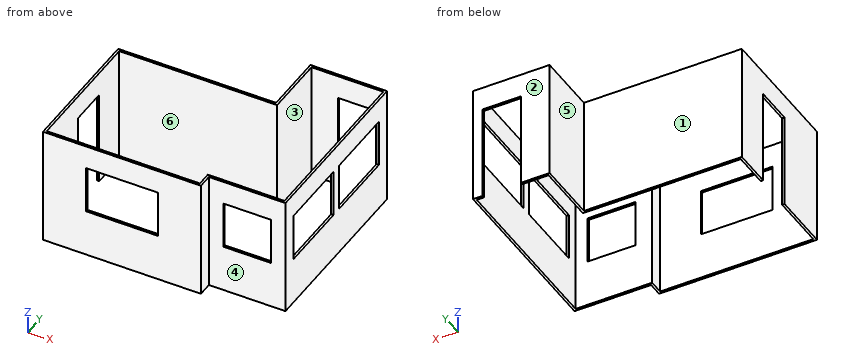
from build123d import *

# Parameters (mm, degrees)
F1_DEPTH  = 63.5
F2_W      = 38.1
F2_H      = 25.4
F3_DEPTH  = 1.27
F4_W      = 25.4
F4_H      = 25.4
F5_DEPTH  = 1.27
F6_W      = 38.1
F6_H      = 25.4
F7_DEPTH  = 1.27
F8_W      = 20.32
F8_H      = 50.8
F9_DEPTH  = 1.27
F10_W     = 20.32
F10_H     = 50.8
F11_DEPTH = 1.27


with BuildPart() as f1:
    # F0 (on Top) → F1 (new body)
    with BuildSketch(Plane.XY):
        Polygon((0, 32.766), (0, 0), (-83.82, 0), (-83.82, -71.628), (0, -71.628), (0, -64.008), (40.64, -64.008), (40.64, 32.766), align=None)
        Polygon((1.27, -1.27), (1.27, 31.496), (39.37, 31.496), (39.37, -62.738), (-1.27, -62.738), (-1.27, -70.358), (-82.55, -70.358), (-82.55, -1.27), align=None, mode=Mode.SUBTRACT)
    extrude(amount=F1_DEPTH)

    # F2 (on face) → F3 (cut)
    with BuildSketch(Plane.XZ.offset(71.628)):
        with Locations((-41.91, 38.1)):
            Rectangle(F2_W, F2_H)
    extrude(amount=-F3_DEPTH, mode=Mode.SUBTRACT)

    # F4 (on face) → F5 (cut)
    with BuildSketch(Plane.XZ.offset(64.008)):
        with Locations((20.32, 38.1)):
            Rectangle(F4_W, F4_H)
    extrude(amount=-F5_DEPTH, mode=Mode.SUBTRACT)

    # F6 (on face) → F7 (cut)
    with BuildSketch(Plane.YZ.offset(40.64)):
        with Locations((-37.338, 38.1)):
            Rectangle(F6_W, F6_H)
        with Locations((6.096, 38.1)):
            Rectangle(F6_W, F6_H)
    extrude(amount=-F7_DEPTH, mode=Mode.SUBTRACT)

    # F8 (on face) → F9 (cut)
    with BuildSketch(Plane(origin=(0, 32.766, 0), x_dir=(-1, 0, 0), z_dir=(0, 1, 0))):
        with Locations((-25.4, 25.4)):
            Rectangle(F8_W, F8_H)
    extrude(amount=-F9_DEPTH, mode=Mode.SUBTRACT)

    # F10 (on face) → F11 (cut)
    with BuildSketch(Plane(origin=(-83.82, 0, 0), x_dir=(0, -1, 0), z_dir=(-1, 0, 0))):
        with Locations((30.48, 25.4)):
            Rectangle(F10_W, F10_H)
    extrude(amount=-F11_DEPTH, mode=Mode.SUBTRACT)


solid = f1.part
Check sheet for the modelled part. Datum: model origin and axes. Units: mm. Face numbers are marked on the shaded views. A direction names the side the tool comes from. Give positions to 0.01 mm unless a question says otherwise; leave off trailing zeros. Write each loop counter-clockwise with the first axis right and the second up, starting at its lowest first coordinate (ties: lowest second). Pieces come first, ordered by that corner, then holes. Notation, with made-up numbers: (17.25, -32) -> (43.25, -32) arc R7 ccw to (43.25, -21) -> close; hole circle Ø1 at (84, 31). An arc over 180 degrees is marked (long way). Use one line per item in the form item = value. Start each with the question number.
1. Go/stop test with flat-tipped pins: P1, Ø16.5, axis at y = 9.5, z = 36.5, coming from the -X side; P2, Ø8, axis at y = -24.5, z = 31.5, coming from the +X side; P3, Ø19, axis at x = -45.5, z = 28.5, coming from the -Y side; P4, Ø11.5, axis at x = 20, z = 16, coming from the -Y side. Record where each tip stops, or that it passes through.
2. Section check D-D (x = -15.5). Record the cut outline in (y, z).
3. Access from +Z, -Z, +X, -X, +Y, -Y to the whole of each face (thin tool, end or side, straight path). Record for the marked faces 1, 2 and 3.
4. Mould release check, pull along X, two halves, no side actions. Record for the marked faces 4, 5 and 6: pulls with the +X half, pulls with the -X half, needs draft (parallel to the pull), parting line crosses it, or undercut.
5. Section check C-C (z = 22.5). Record the cut outline in (x, y).
6. Thickness scan on line 1 along Y through (x, z) = (-63.5, 29.5); line 2 along X through (y, z) = (20.5, 61.5); line 3 along Y through (x, z) = (4, 4.5). Record the ranges inside material, lowest first. Write a range as from..to.
7. Section check B-B (x = -56). Record the cut outline in (y, z), and give its area (3 significant figures).
8. Section check A-A (y = -26.5). Record the cut outline in (x, z), and give its area (3 significant figures).
Conclusion:
q1.P1 = 0
q1.P2 = through
q1.P3 = -71.63
q1.P4 = -64.01
q2.outline = (-71.63, 0) -> (-70.36, 0) -> (-70.36, 63.5) -> (-71.63, 63.5) -> close; (-1.27, 0) -> (0, 0) -> (0, 63.5) -> (-1.27, 63.5) -> close
q3.face_1 = +Z, -Z, -X, +Y
q3.face_2 = +Z, -Z, +X, -X, +Y
q3.face_3 = +Z, -Z
q4.face_4 = needs draft
q4.face_5 = pulls with the -X half
q4.face_6 = undercut
q5.outline = (-83.82, -71.63) -> (0, -71.63) -> (0, -64.01) -> (40.64, -64.01) -> (40.64, 32.77) -> (35.56, 32.77) -> (35.56, 31.5) -> (39.37, 31.5) -> (39.37, -62.74) -> (-1.27, -62.74) -> (-1.27, -70.36) -> (-82.55, -70.36) -> (-82.55, -40.64) -> (-83.82, -40.64) -> close; (-83.82, -20.32) -> (-82.55, -20.32) -> (-82.55, -1.27) -> (1.27, -1.27) -> (1.27, 31.5) -> (15.24, 31.5) -> (15.24, 32.77) -> (0, 32.77) -> (0, 0) -> (-83.82, 0) -> close
q6.line_1 = -71.63..-70.36, -1.27..0
q6.line_2 = 0..1.27, 39.37..40.64
q6.line_3 = -64.01..-62.74, 31.5..32.77
q7.outline = (-71.63, 0) -> (-70.36, 0) -> (-70.36, 25.4) -> (-71.63, 25.4) -> close; (-71.63, 50.8) -> (-70.36, 50.8) -> (-70.36, 63.5) -> (-71.63, 63.5) -> close; (-1.27, 0) -> (0, 0) -> (0, 63.5) -> (-1.27, 63.5) -> close
q7.area = 129 mm²
q8.outline = (-83.82, 50.8) -> (-82.55, 50.8) -> (-82.55, 63.5) -> (-83.82, 63.5) -> close; (39.37, 0) -> (40.64, 0) -> (40.64, 25.4) -> (39.37, 25.4) -> close; (39.37, 50.8) -> (40.64, 50.8) -> (40.64, 63.5) -> (39.37, 63.5) -> close
q8.area = 64.5 mm²
